```python
from build123d import *

# Parameters (mm, degrees)
F1_DEPTH = 114.3
F2_R     = 12.7
F3_DEPTH = 25.4
F6_DEPTH = 2.032
F7_DEPTH = 25.4


with BuildPart() as f1:
    # F0 (on Front) → F1 (new body)
    with BuildSketch(Plane.XZ):
        with BuildLine():
            Line((10.5614215136, -7), (-10.5966975988, -7))
            ThreePointArc((-10.5966975988, -7), (-10.2701474295, -7.4708815929), (-9.9226886379, -7.9265534878))
            Line((-9.9226886379, -7.9265534878), (9.9226886379, -7.9265534878))
            ThreePointArc((9.9226886379, -7.9265534878), (10.2513617434, -7.4966380736), (10.5614215136, -7.0531110592))
            Line((10.5614215136, -7.0531110592), (10.5614215136, -7))
        make_face()
        with BuildLine():
            ThreePointArc((-9.9226886379, -7.9265534878), (-10.2701474295, -7.4708815929), (-10.5966975988, -7))
            Line((-10.5966975988, -7), (-10.5966975988, -7.9265534878))
            Line((-10.5966975988, -7.9265534878), (-9.9226886379, -7.9265534878))
        make_face()
        with BuildLine():
            Line((9.9226886379, -7.9265534878), (-9.9226886379, -7.9265534878))
            ThreePointArc((-9.9226886379, -7.9265534878), (-7.5775508356, -10.1916987463), (-4.7329799249, -11.7851135349))
            Line((-4.7329799249, -11.7851135349), (-4.7329799249, -10.4623720994))
            Line((-4.7329799249, -10.4623720994), (-3.2759574242, -10.4623720994))
            Line((-3.2759574242, -10.4623720994), (-3.2759574242, -12.2702120175))
            ThreePointArc((-3.2759574242, -12.2702120175), (-0.0620753883, -12.6998482923), (3.1558530074, -12.3016499623))
            Line((3.1558530074, -12.3016499623), (3.1558530074, -10.4598701178))
            Line((3.1558530074, -10.4598701178), (4.5460122637, -10.4598701178))
            Line((4.5460122637, -10.4598701178), (4.5460122637, -11.8584894695))
            ThreePointArc((4.5460122637, -11.8584894695), (7.4967230566, -10.2512995963), (9.9226886379, -7.9265534878))
        make_face()
        with BuildLine():
            Line((10.5966975988, -7), (10.5614215136, -7))
            Line((10.5614215136, -7), (10.5614215136, -7.0531110592))
            ThreePointArc((10.5614215136, -7.0531110592), (10.5790928859, -7.026577667), (10.5966975988, -7))
        make_face()
        with BuildLine():
            ThreePointArc((10.5614215136, -7.0531110592), (10.2513617434, -7.4966380736), (9.9226886379, -7.9265534878))
            Line((9.9226886379, -7.9265534878), (10.5614215136, -7.9265534878))
            Line((10.5614215136, -7.9265534878), (10.5614215136, -7.0531110592))
        make_face()
    extrude(amount=F1_DEPTH)

    # F2 (on face) → F3 (join)
    with BuildSketch(Plane.XZ.offset(114.3)):
        Circle(F2_R)
        Polygon((-3.6490469896, 3.6490469896), (0, 5.1605317424), (3.6490469896, 3.6490469896), (5.1605317424, 0), (3.6490469896, -3.6490469896), (0, -5.1605317424), (-3.6490469896, -3.6490469896), (-5.1605317424, 0), align=None, mode=Mode.SUBTRACT)
    extrude(amount=F3_DEPTH)

    # F4: F1 across face


with BuildPart() as f1_1:
    add(f1.part)
    add(f1.part.mirror(Plane(origin=(0.0015510549, 0, -9.2088295832), x_dir=(1, 0, 0), z_dir=(0, 1, 0))))

    # F5 (on face) → F6 (cut)
    with BuildSketch(Plane.XY.offset(-7)):
        Polygon((10.5966975988, 56.0314431787), (-10.5966975988, 56.0314431787), (-10.5966975988, -58.7317496538), (10.5966975988, -58.7317496538), (10.5966975988, 0), align=None)
    extrude(amount=-F6_DEPTH, mode=Mode.SUBTRACT)

    # F2 (on face) → F7 (join)
    with BuildSketch(Plane.XZ.offset(114.3)):
        Circle(F2_R)
        Polygon((-3.6490469896, 3.6490469896), (0, 5.1605317424), (3.6490469896, 3.6490469896), (5.1605317424, 0), (3.6490469896, -3.6490469896), (0, -5.1605317424), (-3.6490469896, -3.6490469896), (-5.1605317424, 0), align=None, mode=Mode.SUBTRACT)
    extrude(amount=F7_DEPTH)


solid = f1_1.part
```
Model file for the job. Use its own axes, mm. Give positions to 0.01 mm unless a question says otherwise; leave off trailing zeros. Loops run counter-clockwise (first coordinate to the right, second up) from the corner with the lowest first, then second, coordinate; pieces in that order, holes last. Notation, with made-up numbers: (40, 84.25) - (64, 84.25) arc R16 cw to (64, 101.25) - close; hole circle Ø7 at (58, -27). An arc over 180 degrees is marked (long way). One line per item, written item: value. Start each with the question number.
1. Probe L1, parallel to Y at x = 3, z = 9.5; L2, parallel to Z at x = 0.75, y = -65; L3, parallel to Z at x = 7, y = -96. List the from-to ranges inside material, lowest first. Write a range as from..to.
2. Pull direction Y, two halves, no side cores. Call faces 1 (the flat face through (5.5, -139.7, 0.2)), 2 (the flat face through (5.5, 139.7, 0.2)), 3 (the flat face through (0, 85, -7)): pulls with the +Y half, pulls with the -Y half, needs draft (parallel to the pull), parting line crosses it, or undercut.
3. Slice it at A-A (z = 8.25). List the corners of the cut face in (x, y).
4. Pin check, flat tips, straight feed: pin 1 (5 mm diameter, centred on x = -1.5, z = -4, fed in from +Y); pin 2 (1.5 mm diameter, centred on y = 72.5, z = -12, fed in from +X); pin 3 (1.5 mm diameter, centred on y = 41.5, z = -11, fed in from -X); pin 4 (6 mm diameter, centred on x = -9, y = 108, fed in from +Z). Stop position of each tip, or through.
5. Slice it at B-B (y = 15.5). List the corners of the cut face in (x, z).
Solution:
1. L1: y = -139.7..-114.3, 114.3..139.7
1. L2: z = -12.68..-7
1. L3: z = -10.6..-7
2. face 1: pulls with the -Y half
2. face 2: pulls with the +Y half
2. face 3: undercut
3. outline: (-9.66, -139.7) - (9.66, -139.7) - (9.66, -114.3) - (-9.66, -114.3) - close; (-9.66, 114.3) - (9.66, 114.3) - (9.66, 139.7) - (-9.66, 139.7) - close
4. pin 1: stops at y = 139.7
4. pin 2: stops at x = 5.89
4. pin 3: stops at x = -7.5
4. pin 4: stops at z = -7
5. outline: (-8.93, -9.03) arc R12.7 ccw to (-4.73, -11.79) - (-4.73, -10.46) - (-3.28, -10.46) - (-3.28, -12.27) arc R12.7 ccw to (3.16, -12.3) - (3.16, -10.46) - (4.55, -10.46) - (4.55, -11.86) arc R12.7 ccw to (8.93, -9.03) - close
